The model under review builds one solid part; all positions refer to its coordinate system, in mm. Round coordinates to 2 decimals unless told otherwise and drop trailing zeros. Use a Markdown table: item, result. Add a question column.
1. The part is to be moulded in two halves that separate along Y. For faces 1 (the flat face through (50, 0, 18)), 2 (the flat face through (50, 3, -25.601)), 3 (the flat face through (50, 6.35, 18)), say which applies: +Y half, -Y half, draft (parallel to the pull), parting line (faces both ways), or undercut.
2. Insertion check: P1, Ø3, axis at x = 39.09, z = 25.2, coming from the +Y side; P2, Ø8, axis at x = -15, z = -2.5, coming from the -Y side. Each pin has a flat end and moves straight along its axis. Give the tip position at first contact, or say it passes through.
3. Consider section A-A on y = 2. Count the separate pieces of the cut face and the enclosed holes in it, then the cut area to 3 significant figures.
4. To check wall thickness, follow probe 1 along X at (y, z) = (1, 38); probe 2 along X at (y, z) = (1.25, 53). State the ranges of each line that lie inside material, in increasing order.
from build123d import *

# Parameters (mm, degrees)
SKETCH1_W              = 263.906
SKETCH1_H              = 88.9
BOSS_EXTRUDE1_DEPTH    = 6.35
F_8_32_TAPPED_HOLE2_D  = 3.4544
F_10_24_TAPPED_HOLE1_D = 3.7973
F_8_32_TAPPED_HOLE3_D  = 3.4544


with BuildPart() as part:
    # Sketch1 → Boss-Extrude1 (new body)
    with BuildSketch(Plane(origin=(0, 0, 0), x_dir=(1, 0, 0), z_dir=(0, 1, 0))):
        with Locations((51.789802803, -18.848747716)):
            Rectangle(SKETCH1_W, SKETCH1_H)
    extrude(amount=BOSS_EXTRUDE1_DEPTH)

    # #8-32 Tapped Hole2 (through all)
    with Locations(Plane(origin=(0, 6.35, 0), x_dir=(1, 0, 0), z_dir=(0, 1, 0))):
        with Locations((-76.003947197, 16.825552284), (-33.141447197, 16.825552284), (-33.141447197, -8.574447716), (-76.003947197, -8.574447716), (-76.003947197, -29.123047716), (-33.141447197, -29.123047716), (-33.141447197, -54.523047716), (-76.003947197, -54.523047716), (179.583552803, 16.825552284), (179.583552803, -8.574447716), (179.583552803, -29.123047716), (179.583552803, -54.523047716), (136.721052803, -54.523047716), (136.721052803, -29.123047716), (136.721052803, -8.574447716), (136.721052803, 16.825552284)):
            Hole(F_8_32_TAPPED_HOLE2_D / 2)

    # #10-24 Tapped Hole1 (through all)
    with Locations(Plane(origin=(0, 6.35, 0), x_dir=(1, 0, 0), z_dir=(0, 1, 0))):
        with Locations((-16.472697197, 9.726252284), (-16.472697197, -2.973747716), (8.927302803, -2.973747716), (8.927302803, 9.726252284)):
            Hole(F_10_24_TAPPED_HOLE1_D / 2)

    # #8-32 Tapped Hole3 (through all)
    with Locations(Plane(origin=(0, 6.35, 0), x_dir=(1, 0, 0), z_dir=(0, 1, 0))):
        with Locations((39.089802803, -50.598747716), (64.489802803, -50.598747716), (51.789802803, -50.598747716), (77.189802803, -50.598747716), (51.789802803, -37.898747716), (77.189802803, -37.898747716), (51.789802803, -25.198747716), (77.189802803, -25.198747716), (51.789802803, -12.498747716), (77.189802803, -12.498747716), (51.789802803, 0.201252284), (77.189802803, 0.201252284), (51.789802803, 12.901252284), (77.189802803, 12.901252284), (39.089802803, -37.898747716), (64.489802803, -37.898747716), (39.089802803, -25.198747716), (64.489802803, -25.198747716), (39.089802803, -12.498747716), (64.489802803, -12.498747716), (39.089802803, 0.201252284), (64.489802803, 0.201252284), (39.089802803, 12.901252284), (64.489802803, 12.901252284)):
            Hole(F_8_32_TAPPED_HOLE3_D / 2)


solid = part.part
Answer block:
| question | item | result |
|---|---|---|
| 1 | face 1 | -Y half |
| 1 | face 2 | draft |
| 1 | face 3 | +Y half |
| 2 | P1 | through |
| 2 | P2 | y = 0 |
| 3 | separate pieces | 1 |
| 3 | enclosed holes | 44 |
| 3 | area | 23,000 mm^2 |
| 4 | probe 1 | -80.16 to 37.37, 40.81 to 50.07, 53.51 to 62.77, 66.21 to 75.47, 78.91 to 183.74 |
| 4 | probe 2 | -80.16 to -76.82, -75.19 to -33.96, -32.33 to 135.91, 137.54 to 178.77, 180.4 to 183.74 |
